Input: part model. Units: mm. Frame: model coordinates. A direction names the side the tool comes from. Round coordinates to 2 decimals unless told otherwise and drop trailing zeros. Loops run counter-clockwise (first coordinate to the right, second up) from the corner with the lowest first, then second, coordinate; pieces in that order, holes last. Notation, with made-up numbers: (-31, 21.5) -> (7, 21.5) arc R35 cw to (7, 60.5) -> close; hole circle Ø6 at (84.25, 62). An arc over 180 degrees is marked (long way). Answer as a JSON object with one key per item and string values. Group by question number.
Item 1: Material intervals for line 1 (X direction, y = 17, z = 9.5); line 2 (Y direction, x = 88.5, z = 13.5); line 3 (X direction, y = 34, z = -11), sorted ascending. Write a range as [from, to].
Item 2: Section query A-A on y = 17. Return loops of the section in (x, z).
Item 3: Pin query (flat end, axial travel): pin 1 (4 mm diameter, centred on y = 5, z = 10.5, fed in from -X); pin 2 (4 mm diameter, centred on x = 78.5, y = 15.5, fed in from -Z); pin 3 (3.5 mm diameter, centred on x = 99.5, y = 8, fed in from -Z). Return the tip coordinate at first contact, or that it passes through.
Item 4: Section query B-B on y = 6. Return loops of the section in (x, z), and give its area (3 significant figures).
Item 5: Section query C-C on z = 14.5. Return loops of the section in (x, y).
Item 6: Draft query along Z for faces 4 (the flat face through (84, 40, -12)), 5 (the flat face through (105, 6, 18)), 6 (the cylindrical face through (83.854, 21.241, -24.997)). Return one class per face: released by +Z, released by -Z, zero draft, split by the parting line, or undercut.
Item 7: Set-up query: faces 1 (the flat face through (103, 3, -24)), 2 (the flat face through (87.5, 21, 11)), 3 (the flat face through (84.5, 20, 12)). Return all of +Z, -Z, +X, -X, +Y, -Y with unobstructed straight access to the full face (end or side cutting, diameter ignored); none if empty.
Item 8: Section query D-D on x = 104. Return loops of the section in (y, z), and give its area (3 significant figures).
from build123d import *

# Parameters (mm, degrees)
BOSS_EXTRUDE1_DEPTH   = 40
BOSS_EXTRUDE1_2_DEPTH = 40
BOSS_EXTRUDE2_DEPTH   = 10
BOSS_EXTRUDE3_DEPTH   = 3


with BuildPart() as part:
    # Sketch1 → Boss-Extrude1 (new body)
    with BuildSketch(Plane(origin=(0, 0, 0), x_dir=(1, 0, 0), z_dir=(0, 1, 0))):
        with BuildLine():
            Line((87.5, 0), (87.5, -20))
            Line((87.5, -20), (87.5, -23))
            Line((87.5, -23), (84.5, -23))
            Line((84.5, -23), (84.5, 0))
            ThreePointArc((84.5, 0), (81.074511679, 23.815405855), (71.075773822, 45.699938464))
            Line((71.075773822, 45.699938464), (73.599174076, 47.322421486))
            ThreePointArc((73.599174076, 47.322421486), (83.952896709, 24.660923222), (87.5, 0))
        make_face()
    extrude(amount=BOSS_EXTRUDE1_DEPTH)



with BuildPart() as body_2:
    # Sketch1 → Boss-Extrude1 2 (new body)
    with BuildSketch(Plane(origin=(0, 0, 0), x_dir=(1, 0, 0), z_dir=(0, 1, 0))):
        with BuildLine():
            Line((122.5, 0), (122.5, -20))
            Line((122.5, -20), (122.5, -23))
            Line((122.5, -23), (125.5, -23))
            Line((125.5, -23), (125.5, 0))
            ThreePointArc((125.5, 0), (120.412440423, 35.370809879), (105.56224396, 67.873873103))
            Line((105.56224396, 67.873873103), (103.038843706, 66.251390081))
            ThreePointArc((103.038843706, 66.251390081), (117.534055393, 34.525292511), (122.5, 0))
        make_face()
    extrude(amount=BOSS_EXTRUDE1_2_DEPTH)


with BuildPart() as part_1:
    add(part.part)

    add(body_2.part)  # Boss-Extrude2 merges body 2
    # Sketch2 → Boss-Extrude2 (add)
    with BuildSketch(Plane.XZ):
        Polygon((87.5, 23), (122.5, 23), (122.5, 18), (87.482549511, 18), align=None)
    extrude(amount=-BOSS_EXTRUDE2_DEPTH)

    # Sketch3 → Boss-Extrude3 (add)
    with BuildSketch(Plane.XZ):
        with BuildLine():
            Line((73.599174076, -47.322421486), (103.038843706, -66.251390081))
            ThreePointArc((103.038843706, -66.251390081), (117.534055393, -34.525292511), (122.5, 0))
            Line((122.5, 0), (122.5, 18))
            Line((122.5, 18), (87.5, 18))
            Line((87.5, 18), (87.5, 0))
            ThreePointArc((87.5, 0), (83.952896709, -24.660923222), (73.599174076, -47.322421486))
        make_face()
    extrude(amount=-BOSS_EXTRUDE3_DEPTH)


solid = part_1.part
Solved:
{
 "1": {"line 1": "[84.5, 87.5], [122.5, 125.5]", "line 2": "[0, 3]", "line 3": "[83.78, 86.81], [122.01, 125.02]"},
 "2": {"outline": "(71.08, -45.7) -> (73.6, -47.32) arc R87.5 ccw to (87.5, 0) -> (87.5, 23) -> (84.5, 23) -> (84.5, 0) arc R84.5 cw to start; (103.04, -66.25) -> (105.56, -67.87) arc R125.5 ccw to (125.5, 0) -> (125.5, 23) -> (122.5, 23) -> (122.5, 0) arc R122.5 cw to start"},
 "3": {"pin 1": "x = 84.5", "pin 2": "z = -42.47", "pin 3": "z = 18"},
 "4": {"outline": "(71.08, -45.7) -> (73.6, -47.32) arc R87.5 ccw to (87.5, 0) -> (87.5, 18) -> (122.5, 18) -> (122.5, 0) arc R122.5 cw to (103.04, -66.25) -> (105.56, -67.87) arc R125.5 ccw to (125.5, 0) -> (125.5, 23) -> (84.5, 23) -> (84.5, 0) arc R84.5 cw to start", "area": "673 mm²"},
 "5": {"outline": "(84.5, 0) -> (125.5, 0) -> (125.5, 40) -> (122.5, 40) -> (122.5, 3) -> (87.5, 3) -> (87.5, 40) -> (84.5, 40) -> close"},
 "6": {"face 4": "zero draft", "face 5": "undercut", "face 6": "released by -Z"},
 "7": {"face 1": "+Y", "face 2": "-Z, +Y", "face 3": "+Z, -X, +Y, -Y"},
 "8": {"outline": "(0, -66.87) -> (40, -66.87) -> (40, -64.73) -> (3, -64.73) -> (3, 18) -> (10, 18) -> (10, 23) -> (0, 23) -> close", "area": "384 mm²"}
}
